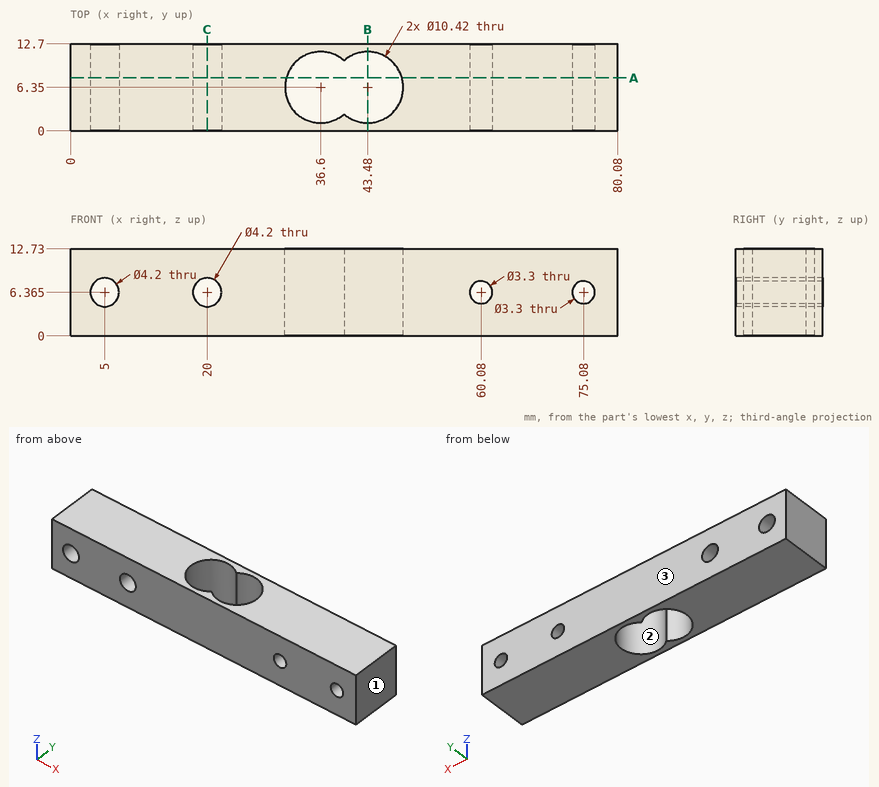
For this review, use the dimensioned drawing (mm, ordinates from the lowest corner) and the shaded views. Round coordinates to 2 decimals unless told otherwise and drop trailing zeros. Loops run counter-clockwise (first coordinate to the right, second up) from the corner with the lowest first, then second, coordinate; pieces in that order, holes last. Notation, with made-up numbers: (85, 77.5) -> (111, 77.5) arc R20 ccw to (111, 106.5) -> close; hole circle Ø8 at (14, 50). An arc over 180 degrees is marked (long way). Write item = value, one per line. Start each with the question number.
Item 1: Take a section at C-C on x = 20. Give the boundary of the cut face in (y, z) (3 decimals).
Item 2: To check wall thickness, follow L1, parallel to Y at x = 43.5, z = 5.75; L2, parallel to X at y = 2.75, z = 6; L3, parallel to X at y = 4.5, z = 7.5. State the ranges of each line that lie inside material, in increasing order.
Item 3: Take a section at B-B on x = 43.48. Give the boundary of the cut face in (y, z), plus the area to 3 significant figures.
Item 4: Take a section at A-A on y = 7.75. Give the boundary of the cut face in (x, z) (3 decimals), plus the area to 3 significant figures.
Item 5: Insertion check: pin 1 (3.5 mm diameter, centred on x = 20, z = 6.365, fed in from -Y). The pin has a flat end and moves straight along its axis. Give the tip position at first contact, or say it passes through.
Item 6: Mouldability with a two-part tool opening along Y and no side actions: class the marked faces 1, 2 and 3 as released by +Y, released by -Y, zero draft, split by the parting line, or undercut.
Result:
q1.outline = (0, 0) -> (12.7, 0) -> (12.7, 4.265) -> (0, 4.265) -> close; (0, 8.465) -> (12.7, 8.465) -> (12.7, 12.73) -> (0, 12.73) -> close
q2.L1 = 0 to 1.14, 11.56 to 12.7
q2.L2 = 0 to 2.93, 7.07 to 17.93, 22.07 to 32.83, 47.25 to 58.47, 61.69 to 73.47, 76.69 to 80.08
q2.L3 = 0 to 3.23, 6.77 to 18.23, 21.77 to 31.73, 48.35 to 58.88, 61.28 to 73.88, 76.28 to 80.08
q3.outline = (0, 0) -> (1.14, 0) -> (1.14, 12.73) -> (0, 12.73) -> close; (11.56, 0) -> (12.7, 0) -> (12.7, 12.73) -> (11.56, 12.73) -> close
q3.area = 29.0 mm²
q4.outline = (0, 0) -> (31.582, 0) -> (31.582, 12.73) -> (0, 12.73) -> close; (48.498, 0) -> (80.08, 0) -> (80.08, 12.73) -> (48.498, 12.73) -> close; hole circle Ø4.2 at (5, 6.365); hole circle Ø4.2 at (20, 6.365); hole circle Ø3.3 at (60.08, 6.365); hole circle Ø3.3 at (75.08, 6.365)
q4.area = 759 mm²
q5.pin_1 = through
q6.face_1 = zero draft
q6.face_2 = undercut
q6.face_3 = released by +Y
